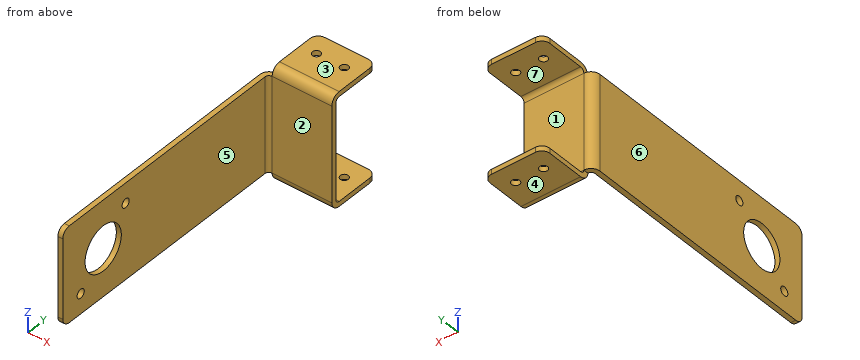
```python
from build123d import *

# Parameters (mm, degrees)
SKETCH1_W               = 38.1
SKETCH1_H               = 60.96
BASE_FLANGE1_DEPTH      = 3.175
EDGE_FLANGE1_DEPTH      = 38.1
EDGE_FLANGE1_BEND_DEPTH = 38.1
EDGE_FLANGE2_DEPTH      = 60.96
SKETCH17_R              = 14.28115
SKETCH17_R_2            = 2.8067
CUT_EXTRUDE1_DEPTH      = 175.607680959
SKETCH18_R              = 2.5527
CUT_EXTRUDE2_DEPTH      = 182.96600596
FILLET1_R               = 5.08


# Sheet-metal steps are written as plain solids
with BuildPart() as part:
    # Sketch1 → Base-Flange1 (new body)
    with BuildSketch(Plane(origin=(0, 0, 0), x_dir=(1, 0, 0), z_dir=(0, 1, 0))):
        Rectangle(SKETCH1_W, SKETCH1_H)
    extrude(amount=-BASE_FLANGE1_DEPTH)

    # Edge-Flange1 section (across the edge) → Edge-Flange1 (add)
    with BuildSketch(Plane(origin=(-19.05, 0, 33.02), x_dir=(0, 0, -1), z_dir=(1, 0, 0))):
        with BuildLine():
            Line((-3.175, 2.54), (-3.175, 31.877))
            Line((-3.175, 31.877), (0, 31.877))
            Line((0, 31.877), (0, 2.54))
            ThreePointArc((0, 2.54), (0.743948776, 0.743948776), (2.54, 0))
            Line((2.54, 0), (2.54, -3.175))
            ThreePointArc((2.54, -3.175), (-1.501115254, -1.501115254), (-3.175, 2.54))
        make_face()
    extrude(amount=EDGE_FLANGE1_DEPTH)

    # Edge-Flange1 section 2 (across the edge) → Edge-Flange1 bend (add)
    with BuildSketch(Plane(origin=(19.05, 0, -33.02), x_dir=(0, 0, 1), z_dir=(-1, 0, 0))):
        with BuildLine():
            Line((-3.175, 2.54), (-3.175, 31.877))
            Line((-3.175, 31.877), (0, 31.877))
            Line((0, 31.877), (0, 2.54))
            ThreePointArc((0, 2.54), (0.743948776, 0.743948776), (2.54, 0))
            Line((2.54, 0), (2.54, -3.175))
            ThreePointArc((2.54, -3.175), (-1.501115254, -1.501115254), (-3.175, 2.54))
        make_face()
    extrude(amount=EDGE_FLANGE1_BEND_DEPTH)

    # Edge-Flange2 section (across the edge) → Edge-Flange2 (add)
    with BuildSketch(Plane(origin=(-21.59, -3.175, 30.48), x_dir=(1, 0, 0), z_dir=(0, 0, -1))):
        with BuildLine():
            Line((-3.175, 2.54), (-3.175, 161.925))
            Line((-3.175, 161.925), (0, 161.925))
            Line((0, 161.925), (0, 2.54))
            ThreePointArc((0, 2.54), (0.743948776, 0.743948776), (2.54, 0))
            Line((2.54, 0), (2.54, -3.175))
            ThreePointArc((2.54, -3.175), (-1.501115254, -1.501115254), (-3.175, 2.54))
        make_face()
    extrude(amount=EDGE_FLANGE2_DEPTH)

    # Sketch17 → Cut-Extrude1 (cut, through all)
    with BuildSketch(Plane.ZY.offset(24.765)):
        with Locations(Location((0, -133.2738, 0), (0, 0, 270))):
            Circle(SKETCH17_R)
        with Locations(Location((-17.7292, -151.003, 0), (0, 0, 270))):
            Circle(SKETCH17_R_2)
        with Locations(Location((17.7292, -115.5446, 0), (0, 0, 270))):
            Circle(SKETCH17_R_2)
    extrude(amount=-CUT_EXTRUDE1_DEPTH, mode=Mode.SUBTRACT)

    # Sketch18 → Cut-Extrude2 (cut, through all)
    with BuildSketch(Plane.XY.offset(36.195)):
        with Locations((8.89, 19.177)):
            Circle(SKETCH18_R)
        with Locations((-8.89, 19.177)):
            Circle(SKETCH18_R)
    extrude(amount=-CUT_EXTRUDE2_DEPTH, mode=Mode.SUBTRACT)

    # Fillet1
    fillet1_edges = [part.edges().sort_by_distance(p)[0] for p in [
        (-19.05, 31.877, 34.6075),
        (19.05, 31.877, 34.6075),
        (19.05, 31.877, -34.6075),
        (-19.05, 31.877, -34.6075),
        (-23.1775, -165.1, 30.48),
        (-23.1775, -165.1, -30.48),
    ]]
    fillet(fillet1_edges, radius=FILLET1_R)


solid = part.part
```
The model under review builds one solid part; all positions refer to its coordinate system, in mm. Face numbers are marked on the shaded views. A direction names the side the tool comes from. Coordinates: 2 decimals unless noted, no trailing zeros. Order: outer loops, then holes, each group sorted by start corner. A loop starts at its lowest first (then second) coordinate and runs counter-clockwise, first axis right, second up. Notation, with made-up numbers: (13.25, 35.25) -> (25.25, 35.25) arc R35 ccw to (25.25, 70.25) -> close; hole circle Ø7 at (72, -7.5). An arc over 180 degrees is marked (long way). Answer in a Markdown table with one row per item. Add a question column.
Item 1: We need section A-A on x = 8.89. Write out the cut boundary in (y, z) (3 decimals), plus the area to 3 significant figures.
Item 2: We need section D-D on z = 28. Write out the cut boundary in (x, y) (3 decimals).
Item 3: Mouldability with a two-part tool opening along Z and no side actions: class the marked faces 1, 2, 3 and 4 as +Z half, -Z half, draft (parallel to the pull), parting line (faces both ways), or undercut.
Item 4: To check wall thickness, follow probe 1 along Z at (x, y) = (12.5, 4.5) (3 decimals); probe 2 along Y at (x, z) = (8, 1) (3 decimals); probe 3 along X at (y, z) = (-71, 23.5) (3 decimals). State the ranges of each line that lie inside material, in increasing order.
Item 5: We need section B-B on z = 0. Write out the cut boundary in (x, y) (3 decimals), plus the area to 3 significant figures.
Item 6: We need section C-C on y = -121. Write out the cut boundary in (x, z) (3 decimals), plus the area to 3 significant figures.
Item 7: Machinability: for the marked faces 5, 6 and 7, which of the approach directions +Z, -Z, +X, -X, +Y, -Y give a long, thin tool a straight path to every point of the face, cutting with its end or side? Answer none if there is none.
Item 8: Clearance check with flat-ended pins moving along their axes: pin 1 (10 mm diameter, centred on x = -19.5, z = 29, fed in from +Y); pin 2 (10 mm diameter, centred on x = -7, z = -21, fed in from -Y) (3 decimals); pin 3 (6.5 mm diameter, centred on x = -22, y = -80, fed in from -Z). State where each tip first meets the part, or that it passes through.
Final values:
| question | item | result |
|---|---|---|
| 1 | outline | (-3.175, -30.48) arc R5.715 ccw to (2.54, -36.195) -> (16.624, -36.195) -> (16.624, -33.02) -> (2.54, -33.02) arc R2.54 cw to (0, -30.48) -> (0, 30.48) arc R2.54 cw to (2.54, 33.02) -> (16.624, 33.02) -> (16.624, 36.195) -> (2.54, 36.195) arc R5.715 ccw to (-3.175, 30.48) -> close; (21.73, -36.195) -> (31.877, -36.195) -> (31.877, -33.02) -> (21.73, -33.02) -> close; (21.73, 33.02) -> (31.877, 33.02) -> (31.877, 36.195) -> (21.73, 36.195) -> close |
| 1 | area | 389 mm2 |
| 2 | outline | (-24.765, -164.384) -> (-21.59, -164.384) -> (-21.59, -5.715) arc R2.54 cw to (-19.05, -3.175) -> (19.05, -3.175) -> (19.05, 0) -> (-19.05, 0) arc R5.715 ccw to (-24.765, -5.715) -> close |
| 3 | face 1 | undercut |
| 3 | face 2 | draft |
| 3 | face 3 | +Z half |
| 3 | face 4 | -Z half |
| 4 | probe 1 | z = -36.195 to -33.02, 33.02 to 36.195 |
| 4 | probe 2 | y = -3.175 to 0 |
| 4 | probe 3 | x = -24.765 to -21.59 |
| 5 | outline | (-24.765, -165.1) -> (-21.59, -165.1) -> (-21.59, -147.555) -> (-24.765, -147.555) -> close; (-24.765, -118.993) -> (-21.59, -118.993) -> (-21.59, -5.715) arc R2.54 cw to (-19.05, -3.175) -> (19.05, -3.175) -> (19.05, 0) -> (-19.05, 0) arc R5.715 ccw to (-24.765, -5.715) -> close |
| 5 | area | 557 mm2 |
| 6 | outline | (-24.765, -30.48) -> (-21.59, -30.48) -> (-21.59, -7.301) -> (-24.765, -7.301) -> close; (-24.765, 7.301) -> (-21.59, 7.301) -> (-21.59, 30.48) -> (-24.765, 30.48) -> close |
| 6 | area | 147 mm2 |
| 7 | face 5 | +Z, -Z, +X, -Y |
| 7 | face 6 | +Z, -Z, -X, +Y, -Y |
| 7 | face 7 | +X, -X, +Y |
| 8 | pin 1 | stops at y = 31.19 |
| 8 | pin 2 | stops at y = -3.175 |
| 8 | pin 3 | stops at z = -30.48 |
